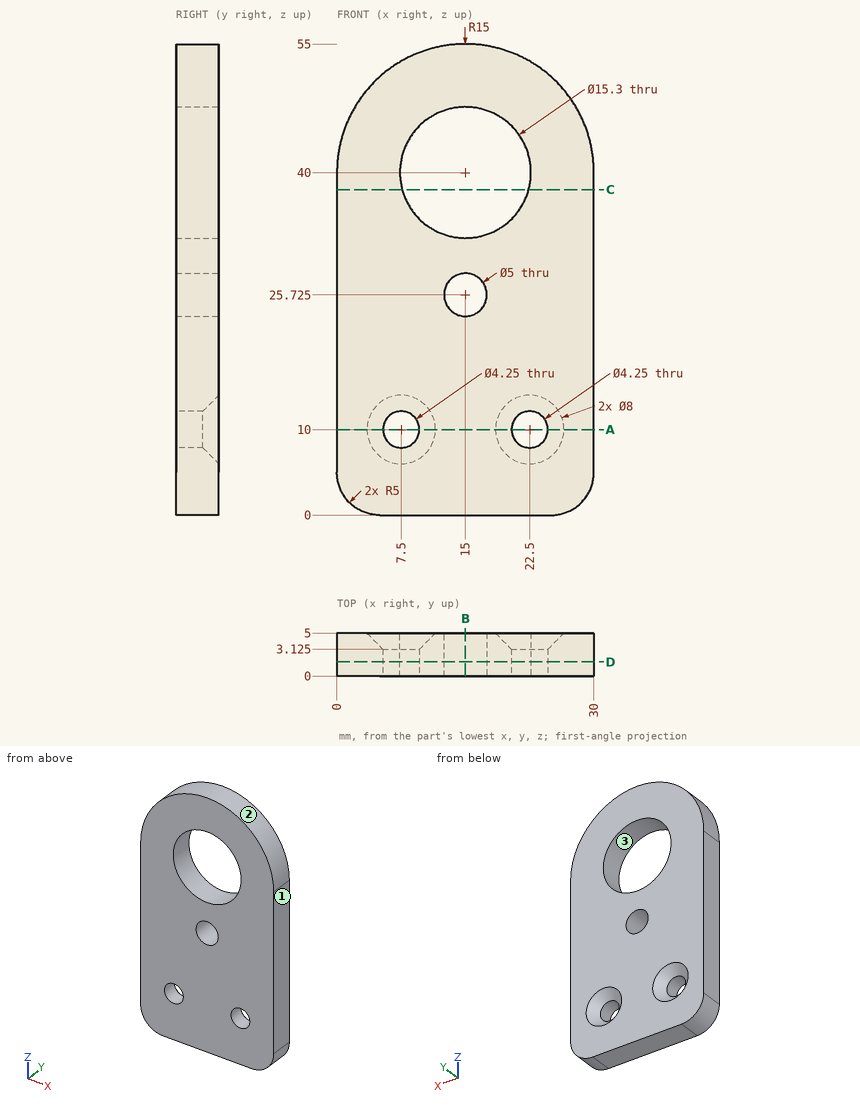
Design review of the part shown in the three views and the two pictorial views. Dimensions are in mm from the part's minimum x, y and z. Give positions to 0.01 mm unless a question says otherwise; leave off trailing zeros. Loops run counter-clockwise (first coordinate to the right, second up) from the corner with the lowest first, then second, coordinate; pieces in that order, holes last. Notation, with made-up numbers: M 83.5,72 L 119.5,72 A23 ccw 119.5,99 Z; hole C -39.5,48 d11. An arc over 180 degrees is marked long. Answer as a JSON object with one key per item and string values. Group by question number.
Q1. Add section C-C on z = 38. Give the boundary of the cut face in (x, y).
Q2. For probe 1 along Z at (x, y) = (15, 3.85) (3 decimals); probe 2 along Z at (x, y) = (13, 4.25) (1 decimal); probe 3 along Z at (x, y) = (19, 0.4), list the stretches that pass through material, from the lowest coordinate up. Write a range as [from, to].
Q3. Insertion check: P1, Ø2, axis at x = 7, y = 4.5, coming from the +Z side; P2, Ø1.5, axis at x = 26.5, y = 4, coming from the +Z side. Each pin has a flat end and moves straight along its axis. Give the tip position at first contact, or say it passes through.
Q4. Mouldability with a two-part tool opening along X and no side actions: class the marked faces 1, 2 and 3 as +X half, -X half, draft (parallel to the pull), parting line (faces both ways), or undercut.
Q5. Add section D-D on y = 1.65. Give the boundary of the cut face in (x, z) (3 decimals).
Q6. Add section B-B on x = 15. Give the boundary of the cut face in (y, z) (3 decimals), and give its area (4 significant figures).
Q7. Add section A-A on z = 10. Give the boundary of the cut face in (x, y) (3 decimals).
Checked values:
{
 "1": {"outline": "M 0,0 L 7.62,0 L 7.62,5 L 0,5 Z; M 22.38,0 L 30,0 L 30,5 L 22.38,5 Z"},
 "2": {"probe 1": "[0, 23.225], [28.225, 32.35], [47.65, 55]", "probe 2": "[0, 24.2], [27.2, 32.6], [47.4, 54.9]", "probe 3": "[0, 33.48], [46.52, 54.46]"},
 "3": {"P1": "z = 53.27", "P2": "z = 50.46"},
 "4": {"face 1": "+X half", "face 2": "parting line", "face 3": "undercut"},
 "5": {"outline": "M 0,5 A5 ccw 5,0 L 25,0 A5 ccw 30,5 L 30,40 A15 ccw 0,40 Z; hole C 7.5,10 d4.25; hole C 15,40 d15.3; hole C 15,25.725 d5; hole C 22.5,10 d4.25"},
 "6": {"outline": "M 0,0 L 5,0 L 5,23.225 L 0,23.225 Z; M 0,28.225 L 5,28.225 L 5,32.35 L 0,32.35 Z; M 0,47.65 L 5,47.65 L 5,55 L 0,55 Z", "area": "173.5 mm²"},
 "7": {"outline": "M 0,0 L 5.375,0 L 5.375,3.125 L 3.5,5 L 0,5 Z; M 9.625,0 L 20.375,0 L 20.375,3.125 L 18.5,5 L 11.5,5 L 9.625,3.125 Z; M 24.625,0 L 30,0 L 30,5 L 26.5,5 L 24.625,3.125 Z"}
}
